The drawing under review shows one solid part. Ordinate dimensions are in mm from its lowest x, y, z. Coordinates: 2 decimals unless noted, no trailing zeros. Write each loop counter-clockwise with the first axis right and the second up, starting at its lowest first coordinate (ties: lowest second). Pieces come first, ordered by that corner, then holes.
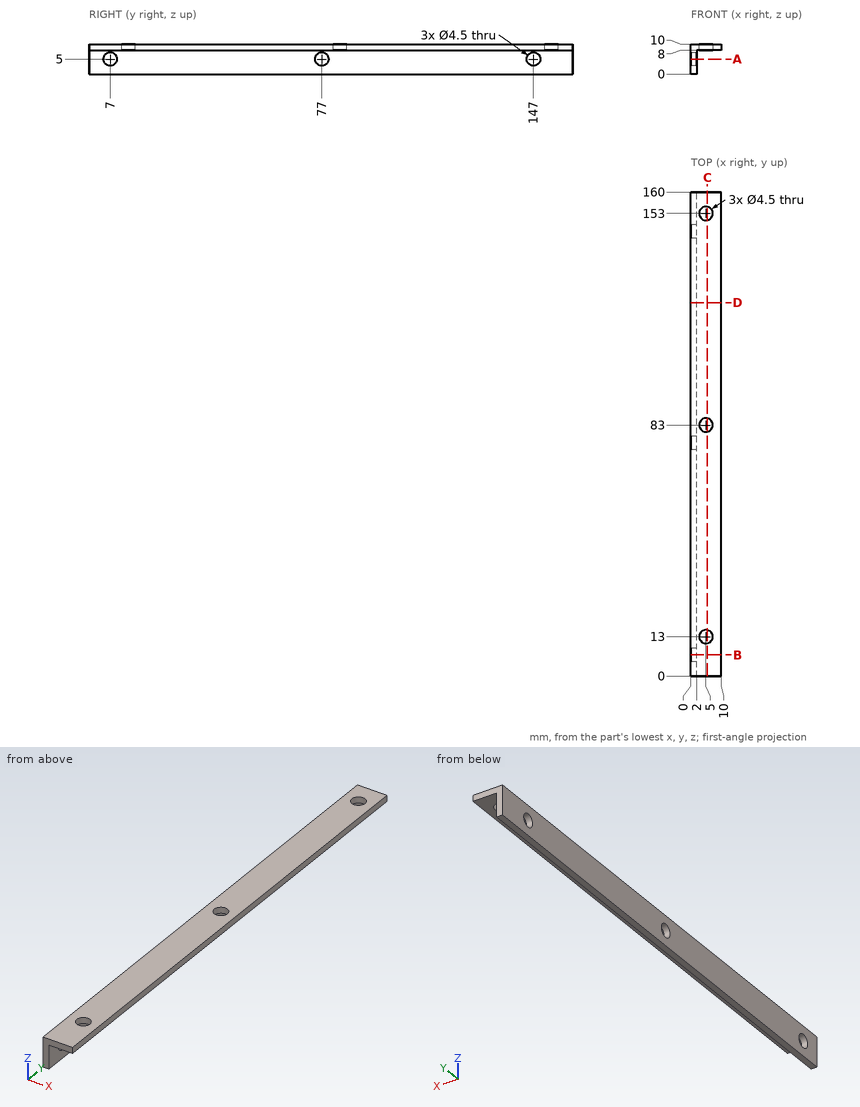
Q1. Clearance check with flat-ended pins moving along their axes: pin 1 Ø5 at (y, z) = (77, 5) entering from +X; pin 2 Ø4 at (x, y) = (7.5, 89) entering from -Z. State where each tip first meets the part, or that it passes through.
Ans:
pin 1: stops at x = 2
pin 2: stops at z = 8
Q2. Add section C-C (x = 5.5). State the section outline as (y, z) points, then the cut area to 3 significant figures.
Ans:
outline: (0, 8) - (10.81, 8) - (10.81, 10) - (0, 10) - close; (15.19, 8) - (80.81, 8) - (80.81, 10) - (15.19, 10) - close; (85.19, 8) - (150.81, 8) - (150.81, 10) - (85.19, 10) - close; (155.19, 8) - (160, 8) - (160, 10) - (155.19, 10) - close
area: 294 mm2
Q3. Add section A-A (z = 5). State the section outline as (x, y) points.
Ans:
outline: (0, 0) - (2, 0) - (2, 4.75) - (0, 4.75) - close; (0, 9.25) - (2, 9.25) - (2, 74.75) - (0, 74.75) - close; (0, 79.25) - (2, 79.25) - (2, 144.75) - (0, 144.75) - close; (0, 149.25) - (2, 149.25) - (2, 160) - (0, 160) - close
Q4. Add section D-D (y = 123.5). State the section outline as (x, z) points, then the cut area to 3 significant figures.
Ans:
outline: (0, 0) - (2, 0) - (2, 8) - (10, 8) - (10, 10) - (0, 10) - close
area: 36.0 mm2
Q5. Add section B-B (y = 7). State the section outline as (x, z) points, then the cut area to 3 significant figures.
Ans:
outline: (0, 0) - (2, 0) - (2, 2.75) - (0, 2.75) - close; (0, 7.25) - (2, 7.25) - (2, 8) - (10, 8) - (10, 10) - (0, 10) - close
area: 27.0 mm2
Q6. For probe 1 along Y at (x, z) = (5, 8.4); probe 2 along Y at (x, z) = (0.7, 5); probe 3 along Z at (x, y) = (1.65, 147), list the stretches that pass through material, from the lowest coordinate up.
Ans:
probe 1: y = 0 to 10.75, 15.25 to 80.75, 85.25 to 150.75, 155.25 to 160
probe 2: y = 0 to 4.75, 9.25 to 74.75, 79.25 to 144.75, 149.25 to 160
probe 3: z = 0 to 2.75, 7.25 to 10
